from build123d import *

# Parameters (mm, degrees)
SKETCH2_W           = 25
SKETCH2_H           = 3
BOSS_EXTRUDE1_DEPTH = 32
CIRPATTERN1_COUNT   = 6
SKETCH5_R           = 6
BOSS_EXTRUDE2_DEPTH = 32
AXLEHOLE_DEPTH      = 53.191951405
FILLET1_R           = 2


with BuildPart() as part:
    # Sketch1 → Revolve1 (revolve)
    with BuildSketch(Plane.XZ, mode=Mode.PRIVATE) as revolve1_sk:
        with BuildLine():
            Line((25, 0), (28, 0))
            Line((28, 0), (28, 1.5))
            Line((28, 1.5), (26.8, 1.5))
            Line((26.8, 1.5), (26.8, 4.5))
            Line((26.8, 4.5), (28, 4.5))
            Line((28, 4.5), (28, 6))
            Line((28, 6), (26.8, 6))
            Line((26.8, 6), (26.8, 28))
            Line((26.8, 28), (28, 28))
            Line((28, 28), (28, 29.5))
            Line((28, 29.5), (26.8, 29.5))
            Line((26.8, 29.5), (26.8, 32.5))
            Line((26.8, 32.5), (28, 32.5))
            Line((28, 32.5), (28, 33.999996833))
            Line((28, 33.999996833), (27, 33.999996833))
            ThreePointArc((27, 33.999996833), (25.585786438, 33.414213562), (25, 32))
            Line((25, 32), (25, 0))
        make_face()
    revolve(revolve1_sk.sketch.rotate(Axis((0, 0, 34), (0, 0, -1)), 180), axis=Axis((0, 0, 34), (0, 0, -1)))

    # Sketch2 → Boss-Extrude1 (add)
    with BuildSketch(Plane.XY):
        with Locations((12.5, 0)):
            Rectangle(SKETCH2_W, SKETCH2_H)
    boss_extrude1 = extrude(amount=BOSS_EXTRUDE1_DEPTH)

    # CirPattern1: Boss-Extrude1 ×6 about axis
    cirpattern1_axis = Axis((0, 0, 0), (0, 0, 1))
    for i in range(1, CIRPATTERN1_COUNT):
        add(boss_extrude1.rotate(cirpattern1_axis, i * 360 / CIRPATTERN1_COUNT))

    # Sketch5 → Boss-Extrude2 (add)
    with BuildSketch(Plane.XY):
        Circle(SKETCH5_R)
    extrude(amount=BOSS_EXTRUDE2_DEPTH)

    # Sketch6 → AxleHole (cut, through all)
    with BuildSketch(Plane.XY):
        Polygon((0, -3.87), (3.351518313, -1.935), (3.351518313, 1.935), (0, 3.87), (-3.351518313, 1.935), (-3.351518313, -1.935), align=None)
    extrude(amount=AXLEHOLE_DEPTH, mode=Mode.SUBTRACT)

    # Fillet1
    # the kernel refuses this fillet: 2 mm, written as the material it adds along each edge
    with BuildSketch(Plane(origin=(-24.954959427, -1.5, 32), x_dir=(0.10620109039764976, -0.9943446728365121, 0), z_dir=(0, 0, -1))) as fillet1_piece_1:
        with BuildLine():
            CenterArc((2.224755634, -1.997850608), FILLET1_R, 87.343441845, 98.752929077)
            Line((0.236066288, -2.210252789), (0.196292501, -2.214500833))
            Line((0.196292501, -2.214500833), (-0.039773787, -0.004248044))
            Line((-0.039773787, -0.004248044), (-0.001853963, 0.039957012))
            ThreePointArc((-0.001853963, 0.039957012), (1.158726893, 0.066867397), (2.319307748, 0.039957012))
            Line((2.319307748, 0.039957012), (2.317453785, 0))
        make_face()
    extrude(amount=32)
    with BuildSketch(Plane(origin=(-13.776517819, -20.861628814, 32), x_dir=(-0.8080272015953212, 0.589145178612228, 0), z_dir=(0, 0, -1)), Plane(origin=(13.776517819, 20.861628814, 32), x_dir=(0.8080272015953204, -0.589145178612229, 0), z_dir=(0, 0, -1)), Plane(origin=(24.954959427, -1.5, 32), x_dir=(-0.10620109039765001, -0.994344672836512, 0), z_dir=(0, 0, -1)), Plane(origin=(-11.178441608, 22.361628814, 32), x_dir=(0.9142282919929711, 0.4051994942242834, 0), z_dir=(0, 0, -1)), Plane(origin=(-24.954959427, 1.5, 32), x_dir=(0.10620109039765026, 0.994344672836512, 0), z_dir=(0, 0, -1))) as fillet1_piece_2:
        with BuildLine():
            CenterArc((2.224755634, 1.997850608), FILLET1_R, 173.903629078, 98.752929077)
            Line((0.236066288, 2.210252789), (0.196292501, 2.214500833))
            Line((0.196292501, 2.214500833), (-0.039773787, 0.004248044))
            Line((-0.039773787, 0.004248044), (-0.001853963, -0.039957012))
            ThreePointArc((-0.001853963, -0.039957012), (1.158726893, -0.066867397), (2.319307748, -0.039957012))
            Line((2.319307748, -0.039957012), (2.317453785, 0))
        make_face()
    extrude(amount=32)
    with BuildSketch(Plane(origin=(-11.178441608, -22.361628814, 32), x_dir=(0.5000000000000002, 0.8660254037844387, 0), z_dir=(0, 0, -1)), Plane(origin=(13.776517819, -20.861628814, 32), x_dir=(-0.5000000000000002, 0.8660254037844387, 0), z_dir=(0, 0, -1)), Plane(origin=(24.954959427, 1.5, 32), x_dir=(-1, 0, 0), z_dir=(0, 0, -1)), Plane(origin=(11.178441608, 22.361628814, 32), x_dir=(-0.4999999999999994, -0.8660254037844389, 0), z_dir=(0, 0, -1)), Plane(origin=(-13.776517819, 20.861628814, 32), x_dir=(0.5000000000000007, -0.8660254037844382, 0), z_dir=(0, 0, -1))) as fillet1_piece_3:
        with BuildLine():
            CenterArc((2.222823584, 2), FILLET1_R, 171.247070923, 98.752929077)
            Line((0.246116119, 2.304347826), (0.20658197, 2.310434783))
            ThreePointArc((0.20658197, 2.310434783), (0.056568819, 1.159275304), (-0.039927935, 0.0024))
            Line((-0.039927935, 0.0024), (0, -0.04))
            Line((0, -0.04), (2.222823584, -0.04))
            Line((2.222823584, -0.04), (2.222823584, 0))
        make_face()
    extrude(amount=32)
    with BuildSketch(Plane(origin=(5.809475019, 1.5, 32), x_dir=(1, 0, 0), z_dir=(0, 0, -1)), Plane(origin=(4.203775615, -4.281152949, 32), x_dir=(0.5000000000000001, -0.8660254037844386, 0), z_dir=(0, 0, -1)), Plane(origin=(1.605699404, 5.781152949, 32), x_dir=(0.4999999999999986, 0.8660254037844394, 0), z_dir=(0, 0, -1)), Plane(origin=(-4.203775615, 4.281152949, 32), x_dir=(-0.5000000000000004, 0.8660254037844384, 0), z_dir=(0, 0, -1)), Plane(origin=(-5.809475019, -1.5, 32), x_dir=(-1, 0, 0), z_dir=(0, 0, -1)), Plane(origin=(-1.605699404, -5.781152949, 32), x_dir=(-0.4999999999999988, -0.8660254037844393, 0), z_dir=(0, 0, -1))) as fillet1_piece_4:
        with BuildLine():
            CenterArc((1.384272266, -2), FILLET1_R, 90, 64.055520228)
            Line((-0.414164556, -1.125), (-0.450133292, -1.1075))
            ThreePointArc((-0.450133292, -1.1075), (-0.216451666, -0.559050695), (-0.038729833, 0.01))
            Line((-0.038729833, 0.01), (0, 0.04))
            Line((0, 0.04), (1.384272266, 0.04))
            Line((1.384272266, 0.04), (1.384272266, 0))
        make_face()
    extrude(amount=32)
    with BuildSketch(Plane(origin=(4.203775615, 4.281152949, 32), x_dir=(0.6399622417657335, -0.7684063567632539, 0), z_dir=(0, 0, -1)), Plane(origin=(5.809475019, -1.5, 32), x_dir=(-0.3454783045035584, -0.9384267372135913, 0), z_dir=(0, 0, -1)), Plane(origin=(-1.605699404, 5.781152949, 32), x_dir=(0.9854405462692932, 0.1700203804503366, 0), z_dir=(0, 0, -1)), Plane(origin=(-5.809475019, 1.5, 32), x_dir=(0.3454783045035597, 0.9384267372135907, 0), z_dir=(0, 0, -1))) as fillet1_piece_5:
        with BuildLine():
            CenterArc((1.398617439, -1.989994715), FILLET1_R, 95.733483793, 64.055520228)
            Line((-0.478236035, -1.299038106), (-0.515773105, -1.285218973))
            Line((-0.515773105, -1.285218973), (-0.037537069, 0.013819132))
            Line((-0.037537069, 0.013819132), (0.00399605, 0.039799894))
            ThreePointArc((0.00399605, 0.039799894), (0.599407474, 0.009984144), (1.194818898, 0.039799894))
            Line((1.194818898, 0.039799894), (1.198814948, 0))
        make_face()
    extrude(amount=32)
    with BuildSketch(Plane(origin=(-4.203775615, -4.281152949, 32), x_dir=(-0.4999999999999996, -0.8660254037844388, 0), z_dir=(0, 0, -1))) as fillet1_piece_6:
        with BuildLine():
            CenterArc((1.384272266, 2), FILLET1_R, 205.944479772, 64.055520228)
            Line((-0.414164556, 1.125), (-0.450133292, 1.1075))
            ThreePointArc((-0.450133292, 1.1075), (-0.216451666, 0.559050695), (-0.038729833, -0.01))
            Line((-0.038729833, -0.01), (0, -0.04))
            Line((0, -0.04), (1.384272266, -0.04))
            Line((1.384272266, -0.04), (1.384272266, 0))
        make_face()
    extrude(amount=32)
    # the kernel refuses this fillet: 2 mm, written as the material it takes off along each edge
    with BuildSketch(Plane(origin=(-0.894300596, -1.45102593, 32), x_dir=(0.8660254037844385, 0.5000000000000003, 0), z_dir=(0.5000000000000003, -0.8660254037844386, 0))) as fillet1_2_piece_1_section:
        with BuildLine():
            CenterArc((FILLET1_R, -FILLET1_R), FILLET1_R, 90, 90)
            Line((0, -FILLET1_R), (-FILLET1_R * 0.02, -FILLET1_R))
            Line((-FILLET1_R * 0.02, -FILLET1_R), (-FILLET1_R * 0.02, FILLET1_R * 0.02))
            Line((-FILLET1_R * 0.02, FILLET1_R * 0.02), (FILLET1_R, FILLET1_R * 0.02))
            Line((FILLET1_R, FILLET1_R * 0.02), (FILLET1_R, 0))
        make_face()
    fillet1_2_piece_1 = extrude(amount=29.145484408, mode=Mode.PRIVATE)
    fillet1_2_piece_1 = fillet1_2_piece_1 - Plane(origin=(0, 0, 31.546531325), x_dir=(1, 0, 0), z_dir=(0, 0, -1)) * Cylinder(6, 67, mode=Mode.PRIVATE)
    fillet1_2_piece_1 = fillet1_2_piece_1 & Plane(origin=(0, 0, 31.546531325), x_dir=(-1, 0, 0), z_dir=(0, 0, -1)) * Cylinder(25, 67, mode=Mode.PRIVATE)
    add(fillet1_2_piece_1, mode=Mode.SUBTRACT)


solid = part.part
Design review of the part built by this model. Coordinates are the model's own, in mm. A direction names the side the tool comes from. Give positions to 0.01 mm unless a question says otherwise; leave off trailing zeros. One line per question, with ' | ' between items. Start each with the question number.
(1) For faces 4 (the face through (5.81, -26.163, 31.021)), 5 (the face through (24.234, -2.18, 16.224)), list the 3-axis set-ups (+Z, -Z, +X, -X, +Y, -Y) from which the entire face can be reached by the end or side of a thin tool; tool diameter is ignored.
(2) Draft analysis for pull direction Y (two halves, no side actions). For faces 1 (the face through (21.585, 12.612, 15.776)), 2 (the face through (5.81, -26.163, 3.021)), 3 (the face through (-14.005, -19.898, 16.224)), state which applies: +Y half, -Y half, draft (parallel to the pull), parting line (faces both ways), or undercut.
(3) Insertion check: P1, Ø5, axis at x = -4, y = 21.5, coming from the +Z side; P2, Ø8, axis at x = -12.5, z = 14, coming from the +Y side; P3, Ø2, axis at x = -19, z = 19, coming from the +Y side; P4, Ø4, axis at x = -11.5, z = 25, coming from the -Y side. Each pin has a flat end and moves straight along its axis. Give the tip position at first contact, or say it passes through.
(4) We need section A-A (x = -13.5). State how many separate pieces and enclosed holes the cut face has, and give its area (3 significant figures).
(5) For line 1 (Z direction, x = -20, y = 18); line 2 (Y direction, x = -9, z = 7.5); line 3 (Y direction, x = 7.5, z = 8), list the stretches that pass through material, from the lowest coordinate up.
The answers:
1) face 4: none | face 5: +Z, -Z
2) face 1: undercut | face 2: parting line | face 3: undercut
3) P1: passes through | P2: stops at y = 25.42 | P3: stops at y = 19.86 | P4: stops at y = -25.06
4) separate pieces: 3 | enclosed holes: 0 | area: 338 mm^2
5) line 1: z = 0 to 1.5, 4.5 to 6, 28 to 29.5, 32.5 to 34 | line 2: y = -25.24 to -23.32, -18.59 to -12.59, -1.5 to 1.5, 12.59 to 18.59, 23.32 to 25.24 | line 3: y = -25.73 to -23.85, -15.99 to -9.99, -1.5 to 1.5, 9.99 to 15.99, 23.85 to 25.73
